Read the model definition and answer for the solid it produces. Units are mm, in the model's axes. A direction names the side the tool comes from. Round coordinates to 2 decimals unless told otherwise and drop trailing zeros. Write each loop counter-clockwise with the first axis right and the second up, starting at its lowest first coordinate (ties: lowest second). Pieces come first, ordered by that corner, then holes.
from build123d import *

# Parameters (mm, degrees)
BOSS_EXTRUDE1_DEPTH = 80
CUT_EXTRUDE3_DEPTH  = 74


with BuildPart() as part:
    # Sketch1 → Boss-Extrude1 (new, symmetric)
    with BuildSketch(Plane.XY):
        with BuildLine():
            Line((17.5, 0), (12, 0))
            ThreePointArc((12, 0), (0, 12), (-12, 0))
            Line((-12, 0), (-17.5, 0))
            ThreePointArc((-17.5, 0), (0, 17.5), (17.5, 0))
        make_face()
    extrude(amount=BOSS_EXTRUDE1_DEPTH, both=True)

    # Sketch4 → Cut-Extrude3 (cut, symmetric)
    with BuildSketch(Plane.XY):
        with BuildLine():
            Line((0, 0), (12.374368671, 12.374368671))
            ThreePointArc((12.374368671, 12.374368671), (0, 17.5), (-12.374368671, 12.374368671))
            Line((-12.374368671, 12.374368671), (0, 0))
        make_face()
    extrude(amount=CUT_EXTRUDE3_DEPTH, both=True, mode=Mode.SUBTRACT)


solid = part.part
Q1. Straight lines are drawn through the part: probe 1 along Z at (x, y) = (-3, 15.5); probe 2 along X at (y, z) = (0.75, 17.5); probe 3 along X at (y, z) = (6.75, -52). For each, find the intervals that lie inside material, in ascending order.
Verdict:
probe 1: z = -80 to -74, 74 to 80
probe 2: x = -17.48 to -11.98, 11.98 to 17.48
probe 3: x = -16.15 to -9.92, 9.92 to 16.15
Q2. Section A-A (x = 0) is taken. Determine the outline of the cut face in (y, z), then the cut area to 3 significant figures.
Verdict:
outline: (12, -80) - (17.5, -80) - (17.5, -74) - (12, -74) - close; (12, 74) - (17.5, 74) - (17.5, 80) - (12, 80) - close
area: 66.0 mm2
Q3. Flat-ended cylindrical pins translate along their axes: pin 1 Ø10 at (x, z) = (-7.5, 48.5) entering from +Y; pin 2 Ø1.5 at (y, z) = (11, 28.5) entering from -X; pin 3 Ø1.5 at (y, z) = (2, 11) entering from +X. Find the tip coordinate at first contact, or state that the pin passes through.
Verdict:
pin 1: stops at y = 12.37
pin 2: stops at x = -14.18
pin 3: stops at x = 17.46
Q4. Section C-C (y = 10.25) is taken. Determine the outline of the cut face in (x, z).
Verdict:
outline: (-14.18, -80) - (-6.24, -80) - (-6.24, -74) - (-10.25, -74) - (-10.25, 74) - (-6.24, 74) - (-6.24, 80) - (-14.18, 80) - close; (6.24, -80) - (14.18, -80) - (14.18, 80) - (6.24, 80) - (6.24, 74) - (10.25, 74) - (10.25, -74) - (6.24, -74) - close
Q5. Which of the six approach directions +Z, -Z, +X, -X, +Y, -Y give full straight-line access (tool end or side, diameter ignored) to faces 4 (the flat face through (10, 10, 1)), 5 (the flat face through (-15, 0, 1))?
Verdict:
face 4: +Y
face 5: +Z, -Z, +X, -X, -Y
Q6. Determine the mould class of faces 1 (the flat face through (15, 0, 1)), 2 (the cylindrical face through (-15.344, 8.415, 1.12)), 3 (the flat face through (-10, 10, 1)) for opening direction X: pulls with the +X half, pulls with the -X half, needs draft (parallel to the pull), parting line crosses it, or undercut.
Verdict:
face 1: needs draft
face 2: parting line crosses it
face 3: undercut
Q7. Section B-B (z = 66.5) is taken. Determine the outline of the cut face in (x, y), then the cut area to 3 significant figures.
Verdict:
outline: (-17.5, 0) - (-12, 0) arc R12 cw to (-8.49, 8.49) - (-12.37, 12.37) arc R17.5 ccw to start; (8.49, 8.49) arc R12 cw to (12, 0) - (17.5, 0) arc R17.5 ccw to (12.37, 12.37) - close
area: 127 mm2
Q8. Section D-D (x = 10) is taken. Determine the outline of the cut face in (y, z), then the cut area to 3 significant figures.
Verdict:
outline: (6.63, -80) - (14.36, -80) - (14.36, -74) - (10, -74) - (10, 74) - (14.36, 74) - (14.36, 80) - (6.63, 80) - close
area: 591 mm2
